Build history of the part. All positions in model axes, mm. Face numbers are marked on the shaded views. Coordinates: 2 decimals unless noted, no trailing zeros. Order: outer loops, then holes, each group sorted by start corner. A loop starts at its lowest first (then second) coordinate and runs counter-clockwise, first axis right, second up. Notation, with made-up numbers: (-29, -30) - (2, -30) arc R34 cw to (2, 4) - close; hole circle Ø6 at (28, 84.5). An arc over 180 degrees is marked (long way). One line per item, written item: value.
from build123d import *

# Parameters (mm, degrees)
ESQUISSE1_R             = 1.5
ESQUISSE1_R_2           = 1
BOSS_EXTRU_1_DEPTH      = 5
ENL_V_MAT_EXTRU_1_DEPTH = 5
ESQUISSE5_W             = 5
ESQUISSE5_H             = 12
BOSS_EXTRU_2_DEPTH      = 30
CONG_3_START            = -20.022088667
CONG_3_DEPTH            = 7.142932423
CONG_3_START_2          = -12.879156244
CONG_3_2_DEPTH          = 25.906077345
CONG_3_3_OUTLINE_R      = 1
CONG_3_3_OUTLINE_R_2    = 1.5
CONG_3_3_DEPTH          = 5
CONG_4_START            = -20.022088667
CONG_4_DEPTH            = 30
CONG_4_2_DEPTH          = 7.14293242
CONG_4_START_2          = -12.879156247
CONG_4_3_DEPTH          = 25.906077346
CONG_4_4_OUTLINE_R      = 1
CONG_4_4_OUTLINE_R_2    = 1.5
CONG_4_4_DEPTH          = 5
ENL_V_START             = -27
ENL_V_MAT_EXTRU_2_DEPTH = 27
ENL_V_MAT_EXTRU_3_DEPTH = 30


with BuildPart() as part:
    # Esquisse1 → Boss.-Extru.1 (new body)
    with BuildSketch(Plane.XY):
        with BuildLine():
            Line((-22.897983435, -17.234182679), (14.345633901, 0.026586982))
            add(Edge.make_bspline(
                [(14.345633901, 0.026586982), (16.492281726, 0.559482648), (18.723148816, 0.988675042), (21.041646725, 1.309858226)],
                knots=[0, 0, 0, 0, 0.141370549, 0.141370549, 0.141370549, 0.141370549], degree=3))
            ThreePointArc((21.041646725, 1.309858226), (27.202255265, 12.598116604), (14.60702072, 15.193871131))
            add(Edge.make_bspline(
                [(14.60702072, 15.193871131), (12.863335774, 13.632412198), (11.093879733, 12.207631723), (9.299732983, 10.914143371)],
                knots=[0, 0, 0, 0, 0.141370549, 0.141370549, 0.141370549, 0.141370549], degree=3))
            Line((9.299732983, 10.914143371), (-27.943884355, -6.346626291))
            Line((-27.943884355, -6.346626291), (-22.897983435, -17.234182679))
        make_face()
        with Locations((19.943884355, 9.234182671)):
            Circle(ESQUISSE1_R, mode=Mode.SUBTRACT)
        with Locations((10.553366977, 4.882093131)):
            Circle(ESQUISSE1_R_2, mode=Mode.SUBTRACT)
    extrude(amount=BOSS_EXTRU_1_DEPTH)

    # Esquisse2 → Enlèv. mat.-Extru.1 (cut)
    with BuildSketch(Plane.XY.offset(5)):
        Polygon((-53.781292167, 9.271840667), (-26.364947587, 9.271840667), (-1.521431989, -44.333091582), (-53.781292167, -44.333091582), align=None)
    extrude(amount=-ENL_V_MAT_EXTRU_1_DEPTH, mode=Mode.SUBTRACT)

    # Esquisse5 → Boss.-Extru.2 (add)
    with BuildSketch(Plane(origin=(-18.165968268, -8.419122963, 0), x_dir=(0, 0, 1), z_dir=(-0.9072963650485315, -0.42049174304583187, 0))):
        with Locations((7.5, -0.008098332)):
            Rectangle(ESQUISSE5_W, ESQUISSE5_H)
    extrude(amount=-BOSS_EXTRU_2_DEPTH)

    # Congé3: read off the stored shape, not the designer's step
    # Congé3 outline → Congé3 (cut)
    with BuildSketch(Plane(origin=(0, 0, 0), x_dir=(-0.4204917430458318, 0.9072963650485315, 0), z_dir=(0.9072963650485315, 0.4204917430458318, 0)).offset(CONG_3_START)):
        with BuildLine():
            Line((5.991901676, 0), (5.991901676, 5))
            ThreePointArc((5.991901676, 5), (4.527435582, 1.464466094), (0.991901676, 0))
            Line((0.991901676, 0), (5.991901676, 0))
        make_face()
    extrude(amount=CONG_3_DEPTH, mode=Mode.SUBTRACT)

    # Cong_3 2 outline → Cong_3 2 (cut)
    with BuildSketch(Plane(origin=(0, 0, 0), x_dir=(-0.4204917430458318, 0.9072963650485315, 0), z_dir=(0.9072963650485315, 0.4204917430458318, 0)).offset(CONG_3_START_2)):
        with BuildLine():
            Line((5.991901676, 0), (5.991901676, 5))
            ThreePointArc((5.991901676, 5), (4.527435582, 1.464466094), (0.991901676, 0))
            Line((0.991901676, 0), (5.991901676, 0))
        make_face()
    extrude(amount=CONG_3_2_DEPTH, mode=Mode.SUBTRACT)

    # Cong_3 3 outline → Cong_3 3 (add)
    with BuildSketch(Plane.XY):
        with BuildLine():
            Line((-18.583054733, -7.519174178), (-15.639612528, -13.870248741))
            Line((-15.639612528, -13.870248741), (14.345633901, 0.026586982))
            add(Edge.make_bspline(
                [(14.345633901, 0.026586982), (16.492281726, 0.559482648), (18.723148816, 0.988675042), (21.041646725, 1.309858226)],
                knots=[0, 0, 0, 0, 0.141370549, 0.141370549, 0.141370549, 0.141370549], degree=3))
            ThreePointArc((21.041646725, 1.309858226), (27.202255265, 12.598116604), (14.60702072, 15.193871131))
            add(Edge.make_bspline(
                [(14.60702072, 15.193871131), (12.863335774, 13.632412198), (11.093879733, 12.207631723), (9.299732983, 10.914143371), (2.165722649, 5.77088557), (-4.968287685, 0.62762777), (-12.102298019, -4.515630031)],
                knots=[0, 0, 0, 0, 0.141370549, 0.141370549, 0.141370549, 0.703497896, 0.703497896, 0.703497896, 0.703497896], degree=3))
            Line((-12.102298019, -4.515630031), (-18.583054733, -7.519174178))
        make_face()
        with Locations((10.553366977, 4.882093131)):
            Circle(CONG_3_3_OUTLINE_R, mode=Mode.SUBTRACT)
        with Locations((19.943884355, 9.234182671)):
            Circle(CONG_3_3_OUTLINE_R_2, mode=Mode.SUBTRACT)
    extrude(amount=CONG_3_3_DEPTH)

    # Congé4: read off the stored shape, not the designer's step
    # Congé4 outline → Congé4 (cut)
    with BuildSketch(Plane(origin=(0, 0, 0), x_dir=(-0.4204917430458318, 0.9072963650485315, 0), z_dir=(0.9072963650485315, 0.4204917430458318, 0)).offset(CONG_4_START)):
        with BuildLine():
            ThreePointArc((-6.008098332, 5), (-4.543632238, 8.535533906), (-1.008098332, 10))
            Line((-1.008098332, 10), (-6.008098332, 10))
            Line((-6.008098332, 10), (-6.008098332, 5))
        make_face()
        with BuildLine():
            ThreePointArc((0.991901676, 10), (4.527435582, 8.535533906), (5.991901676, 5))
            Line((5.991901676, 5), (5.991901676, 10))
            Line((5.991901676, 10), (0.991901676, 10))
        make_face()
    extrude(amount=CONG_4_DEPTH, mode=Mode.SUBTRACT)

    # Cong_4 2 outline → Cong_4 2 (cut)
    with BuildSketch(Plane(origin=(0, 0, 0), x_dir=(-0.4204917430458318, 0.9072963650485315, 0), z_dir=(0.9072963650485315, 0.4204917430458318, 0)).offset(CONG_4_START)):
        with BuildLine():
            ThreePointArc((-1.008098332, 0), (-4.543632238, 1.464466094), (-6.008098332, 5))
            Line((-6.008098332, 5), (-6.008098332, 0))
            Line((-6.008098332, 0), (-1.008098332, 0))
        make_face()
    extrude(amount=CONG_4_2_DEPTH, mode=Mode.SUBTRACT)

    # Cong_4 3 outline → Cong_4 3 (cut)
    with BuildSketch(Plane(origin=(0, 0, 0), x_dir=(-0.42049174304583214, 0.9072963650485313, 0), z_dir=(0.9072963650485314, 0.42049174304583214, 0)).offset(CONG_4_START_2)):
        with BuildLine():
            ThreePointArc((-1.008098332, 0), (-4.543632238, 1.464466094), (-6.008098332, 5))
            Line((-6.008098332, 5), (-6.008098332, 0))
            Line((-6.008098332, 0), (-1.008098332, 0))
        make_face()
    extrude(amount=CONG_4_3_DEPTH, mode=Mode.SUBTRACT)

    # Cong_4 4 outline → Cong_4 4 (add)
    with BuildSketch(Plane.XY):
        with BuildLine():
            Line((-17.742071243, -9.333766915), (-11.261314532, -6.330222769))
            add(Edge.make_bspline(
                [(-11.261314532, -6.330222769), (-2.725665054, -4.211286186), (5.809984423, -2.092349602), (14.345633901, 0.026586982), (16.492281726, 0.559482648), (18.723148816, 0.988675042), (21.041646725, 1.309858226)],
                knots=[-0.562127348, -0.562127348, -0.562127348, -0.562127348, 0, 0, 0, 0.141370549, 0.141370549, 0.141370549, 0.141370549], degree=3))
            ThreePointArc((21.041646725, 1.309858226), (27.202255265, 12.598116604), (14.60702072, 15.193871131))
            add(Edge.make_bspline(
                [(14.60702072, 15.193871131), (12.863335774, 13.632412198), (11.093879733, 12.207631723), (9.299732983, 10.914143371), (2.165722649, 5.77088557), (-4.968287685, 0.62762777), (-12.102298019, -4.515630031)],
                knots=[0, 0, 0, 0, 0.141370549, 0.141370549, 0.141370549, 0.703497896, 0.703497896, 0.703497896, 0.703497896], degree=3))
            Line((-12.102298019, -4.515630031), (-18.583054733, -7.519174178))
            Line((-18.583054733, -7.519174178), (-17.742071243, -9.333766915))
        make_face()
        with Locations((10.553366977, 4.882093131)):
            Circle(CONG_4_4_OUTLINE_R, mode=Mode.SUBTRACT)
        with Locations((19.943884355, 9.234182671)):
            Circle(CONG_4_4_OUTLINE_R_2, mode=Mode.SUBTRACT)
    extrude(amount=CONG_4_4_DEPTH)

    # Esquisse7 → Enlèv. mat.-Extru.2 (cut)
    with BuildSketch(Plane(origin=(9.052922683, 4.195629328, 0), x_dir=(0, 0, -1), z_dir=(0.9072963650485316, 0.42049174304583187, 0)).offset(ENL_V_START)):
        with BuildLine():
            Line((-10, 0.991901676), (-10, -1.008098332))
            ThreePointArc((-10, -1.008098332), (-8.535533906, -4.543632238), (-5, -6.008098332))
            Line((-5, -6.008098332), (-5, 5.991901668))
            ThreePointArc((-5, 5.991901668), (-8.5355339, 4.527435576), (-10, 0.991901676))
        make_face()
    extrude(amount=ENL_V_MAT_EXTRU_2_DEPTH, mode=Mode.SUBTRACT)

    # Esquisse9 → Enlèv. mat.-Extru.3 (cut)
    with BuildSketch(Plane(origin=(-18.165968268, -8.419122963, 0), x_dir=(0, 0, 1), z_dir=(-0.9072963650485315, -0.42049174304583187, 0))):
        Polygon((1.5, -2.028824274), (5, -4.049550216), (8.5, -2.028824274), (8.5, 2.01262761), (5, 4.033353552), (1.5, 2.01262761), align=None)
    extrude(amount=-ENL_V_MAT_EXTRU_3_DEPTH, mode=Mode.SUBTRACT)


solid = part.part
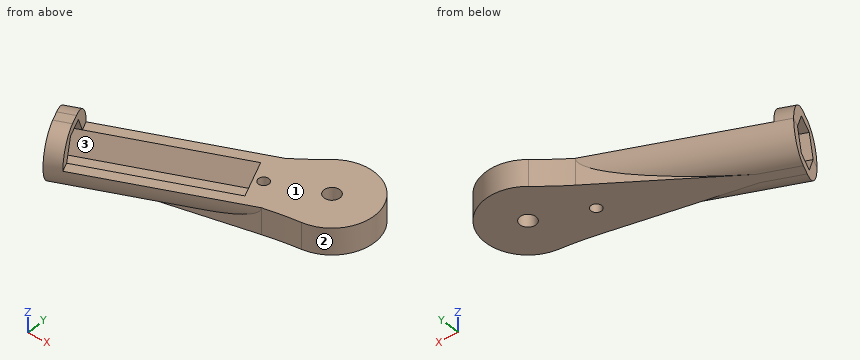
1. Band-saw the part on B-B, the plane z = 4.5. Count the separate pieces of the cut face and the enclosed holes in it, and give its area (3 significant figures).
Values found:
separate pieces: 1
enclosed holes: 2
area: 386 mm2
2. Band-saw the part on A-A, the plane z = 7.5. Give the cut face in (x, y), and give its area (3 significant figures).
Values found:
outline: (-20.4, -3.59) - (-19.26, -6.07) - (-16.53, -4.81) - (-17.68, -2.33) - close; (-17.07, -10.78) - (-15.92, -13.26) - (-13.2, -12) - (-14.35, -9.52) - close
area: 16.4 mm2
3. Band-saw the part on C-C, the plane x = 24. Give the cut face in (y, z), and give its area (3 significant figures).
Values found:
outline: (2.34, 0) - (16.13, 0) - (16.13, 5) - (2.34, 5) - close
area: 69.0 mm2
4. Two-plate mould, pull along X, no slides. Class the marked faces 1, 2 and 3: pulls with the +X half, pulls with the -X half, needs draft (parallel to the pull), parting line crosses it, or undercut.
Values found:
face 1: needs draft
face 2: parting line crosses it
face 3: undercut
5. Probe line 1 along Z through (x, y) = (-16, -7.5); line 2 along Z through (x, y) = (1.5, 1); line 3 along Z through (x, y) = (20, 6). List the from-to ranges inside material, lowest first.
Values found:
line 1: z = 0 to 1.5, 8.5 to 10
line 2: z = 0 to 1.5
line 3: z = 0 to 5
6. Flat gauge pins, fed straight in: P1, Ø1.5, axis at y = -1, z = 3.5, coming from the +X side; P2, Ø10, axis at x = 14, y = -9, coming from the -Z side; P3, Ø18, axis at x = -1.5, y = -5.5, coming from the +Z side; P4, Ø2, axis at x = 15.5, z = 4.5, coming from the +Y side. Where does each tip first touch, or does it go through?
Values found:
P1: stops at x = 13.28
P2: passes through
P3: stops at z = 5
P4: stops at y = 16.45
